```python
from build123d import *

# Parameters (mm, degrees)
SKETCH1_R           = 2
BOSS_EXTRUDE1_DEPTH = 2
CHAMFER1_SIZE       = 0.3
CUT_EXTRUDE1_DEPTH  = 1.5
CHAMFER2_SIZE       = 0.2
SKETCH3_R           = 1
BOSS_EXTRUDE2_DEPTH = 15
CHAMFER3_SIZE       = 0.2


with BuildPart() as part:
    # Sketch1 → Boss-Extrude1 (new body)
    with BuildSketch(Plane(origin=(0, 0, 0), x_dir=(1, 0, 0), z_dir=(0, 1, 0))):
        with Locations(Location((0, 0, 0), (0, 0, 270))):  # turned: the seam where the file's is
            Circle(SKETCH1_R)
    extrude(amount=BOSS_EXTRUDE1_DEPTH)

    # Chamfer1
    chamfer1_edges = [part.edges().sort_by_distance(p)[0] for p in [
        (0, 2, -2),
    ]]
    chamfer(chamfer1_edges, length=CHAMFER1_SIZE)

    # Sketch2 → Cut-Extrude1 (cut)
    with BuildSketch(Plane(origin=(0, 2, 0), x_dir=(1, 0, 0), z_dir=(0, 1, 0))):
        Polygon((1.154700538, 0), (0.577350269, 1), (-0.577350269, 1), (-1.154700538, 0), (-0.577350269, -1), (0.577350269, -1), align=None)
    extrude(amount=-CUT_EXTRUDE1_DEPTH, mode=Mode.SUBTRACT)

    # Chamfer2
    chamfer2_edges = [part.edges().sort_by_distance(p)[0] for p in [
        (0.866025404, 2, 0.5),
        (0.866025404, 2, -0.5),
        (0, 2, -1),
        (-0.866025404, 2, -0.5),
        (-0.866025404, 2, 0.5),
        (0, 2, 1),
    ]]
    chamfer(chamfer2_edges, length=CHAMFER2_SIZE)

    # Sketch3 → Boss-Extrude2 (add)
    with BuildSketch(Plane.XZ):
        with Locations(Location((0, 0, 0), (0, 0, 90))):  # turned: the seam where the file's is
            Circle(SKETCH3_R)
    extrude(amount=BOSS_EXTRUDE2_DEPTH)

    # Chamfer3
    chamfer3_edges = [part.edges().sort_by_distance(p)[0] for p in [
        (0, -15, -1),
    ]]
    chamfer(chamfer3_edges, length=CHAMFER3_SIZE)


solid = part.part
```
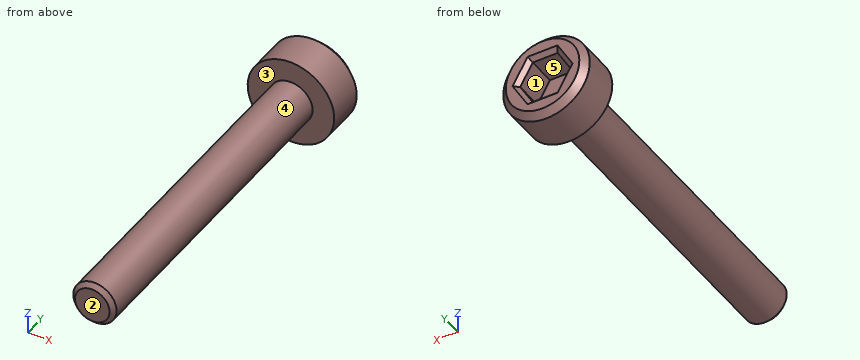
Read the model definition and answer for the solid it produces. Units are mm, in the model's axes. Face numbers are marked on the shaded views. A direction names the side the tool comes from. Give positions to 0.01 mm unless a question says otherwise; leave off trailing zeros. Write each loop counter-clockwise with the first axis right and the second up, starting at its lowest first coordinate (ties: lowest second). Pieces come first, ordered by that corner, then holes. Notation, with made-up numbers: (45, -23.5) - (69, -23.5) arc R19 ccw to (69, -11.5) - close; hole circle Ø6 at (-24.75, 25). An arc over 180 degrees is marked (long way). Write item = value, one per line. Start each with the question number.
Item 1: Find section C-C (y = -13.5). Give the vertices of the cut face in (x, z), then the cut area to 3 significant figures.
Item 2: Find section B-B (x = 0). Give the vertices of the cut face in (y, z), then the cut area to 3 significant figures.
Item 3: The mould has two halves that part along Z. Classify the marked faces 3, 4 and 5: +Z half, -Z half, draft (parallel to the pull), parting line (faces both ways), or undercut.
Item 4: Find the intervals of material crossed by probe 1 along Z at (x, y) = (0.6, -11.5); probe 2 along X at (y, z) = (1, 0.1); probe 3 along Z at (x, y) = (0.4, 0.75), in increasing order. Write a range as [from, to].
Item 5: Find section A-A (y = 1). Give the vertices of the cut face in (x, z), then the cut area to 3 significant figures.
Item 6: A tool of negligible diameter and unlimited length cuts with its end or side. For the marked faces 1 and 2, from which of +Z, -Z, +X, -X, +Y, -Y can it reach the whole face along a straight path? Write none if from no direction.
Response:
q1.outline = circle Ø2 at (0, 0)
q1.area = 3.14 mm²
q2.outline = (-15, -0.8) - (-14.8, -1) - (0, -1) - (0, -2) - (1.7, -2) - (2, -1.7) - (2, -1.2) - (1.8, -1) - (0.5, -1) - (0.5, 1) - (1.8, 1) - (2, 1.2) - (2, 1.7) - (1.7, 2) - (0, 2) - (0, 1) - (-14.8, 1) - (-15, 0.8) - close
q2.area = 34.8 mm²
q3.face_3 = draft
q3.face_4 = parting line
q3.face_5 = undercut
q4.probe_1 = [-0.8, 0.8]
q4.probe_2 = [-2, -1.1], [1.1, 2]
q4.probe_3 = [-1.96, -1], [1, 1.96]
q5.outline = circle Ø4 at (0, 0); hole (-1.15, 0) - (-0.58, -1) - (0.58, -1) - (1.15, 0) - (0.58, 1) - (-0.58, 1) - close
q5.area = 9.10 mm²
q6.face_1 = +Y
q6.face_2 = +Z, -Z, +X, -X, -Y
